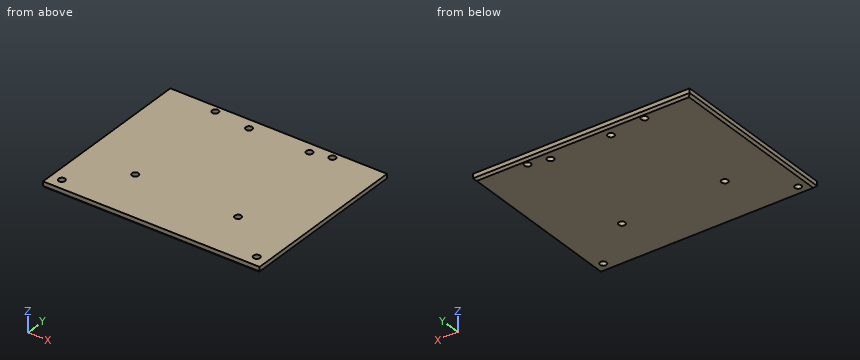
from build123d import *

# Parameters (mm, degrees)
F0_W     = 100
F0_H     = 80
F1_DEPTH = 3
F3_D     = 3
F4_SIZE  = 1
F6_D     = 3


with BuildPart() as f1:
    # F0 (on Top) → F1 (new body)
    with BuildSketch(Plane.XY):
        Rectangle(F0_W, F0_H)
    extrude(amount=F1_DEPTH)

    # F3 (through all)
    with Locations(Plane.XY.offset(3)):
        with Locations((-10, 35), (17.9, 35), (23, -16.8), (-25.2, -15.8)):
            Hole(F3_D / 2)

    # F4
    f4_edges = [f1.edges().sort_by_distance(p)[0] for p in [
        (0, -40, 0),
        (-50, 0, 0),
        (50, 0, 0),
        (0, 40, 0),
    ]]
    chamfer(f4_edges, length=F4_SIZE)

    # F6 (through all)
    with Locations(Plane.XY.offset(3)):
        with Locations((-45, -35), (-27, 37), (27, 37), (45, -35)):
            Hole(F6_D / 2)


solid = f1.part
Input: part model. Units: mm. Frame: model coordinates. Give positions to 0.01 mm unless a question says otherwise; leave off trailing zeros. Order: outer loops, then holes, each group sorted by start corner. A loop starts at its lowest first (then second) coordinate and runs counter-clockwise, first axis right, second up. Notation, with made-up numbers: (-7.75, -1) - (0.25, -1) arc R21 cw to (0.25, 34) - close; hole circle Ø6 at (24, -35). An arc over 180 degrees is marked (long way). Write each question's results on one line, items separated by ' | '.
Item 1: Section A-A (x = -10). Return loops of the section in (y, z).
A:
outline: (-40, 1) - (-39, 0) - (33.5, 0) - (33.5, 3) - (-40, 3) - close; (36.5, 0) - (39, 0) - (40, 1) - (40, 3) - (36.5, 3) - close
Item 2: Material intervals for line 1 along X through (y, z) = (34, 2.1); line 2 along Y through (x, z) = (23, 1.5); line 3 along X through (y, z) = (36, 2.8), sorted ascending.
A:
line 1: x = -50 to -11.12, -8.88 to 16.78, 19.02 to 50 | line 2: y = -40 to -18.3, -15.3 to 40 | line 3: x = -50 to -28.12, -25.88 to -11.12, -8.88 to 16.78, 19.02 to 25.88, 28.12 to 50
Item 3: Contact query for a flat-ended pin moving along its axis: pin 1 Ø2.5 at (x, y) = (-25.2, -15.8) entering from -Z. Output: stop coordinate, or through.
A:
pin 1: passes through
Item 4: Section B-B (y = -35). Return loops of the section in (x, z).
A:
outline: (-50, 1) - (-49, 0) - (-46.5, 0) - (-46.5, 3) - (-50, 3) - close; (-43.5, 0) - (43.5, 0) - (43.5, 3) - (-43.5, 3) - close; (46.5, 0) - (49, 0) - (50, 1) - (50, 3) - (46.5, 3) - close
